Solid Edge part; units mm, degrees
sketch "Sketch1" plane through (0, 0, 0) normal (0, -1, 0) x (1, 0, 0)
  line L0 (-5.4714, -0.2002) -> (36.8286, -0.2002)
  line L1 (36.8286, -0.2002) -> (36.8286, 42.0998)
  line L2 (36.8286, 42.0998) -> (-5.4714, 42.0998)
  line L3 (-5.4714, 42.0998) -> (-5.4714, -0.2002)
extrude "Protrusion1" add sketch "Sketch1" against normal blind 10
sketch "Sketch2" plane through (15.6786, 0, 20.9498) normal (0, -1, 0) x (1, 0, 0)
  circle A0 centre (0, 0) radius 11
extrude "ProtrusiónExtruida_2" add sketch "Sketch2" along normal blind 2
chamfer "Chaflán_2" distance 5 angle 45 4 edges at (36.8286, 5, 42.0998) (36.8286, 5, -0.2002) (-5.4714, 5, -0.2002) (-5.4714, 5, 42.0998)
sketch "Sketch3" plane through (15.6786, -2, 20.9498) normal (0, -1, 0) x (1, 0, 0)
  circle A0 centre (0, 0) radius 4
  circle A1 centre (15.5, 15.5) radius 1.5
  circle A2 centre (-15.5, 15.5) radius 1.5
  circle A3 centre (-15.5, -15.5) radius 1.5
  circle A4 centre (15.5, -15.5) radius 1.5
extrude "VaciadoExtruido_2" cut sketch "Sketch3" against normal blind 7
sketch "Sketch4" plane through (15.6786, 5, 20.9498) normal (0, -1, 0) x (1, 0, 0)
  circle A0 centre (0, 0) radius 2.5
extrude "ProtrusiónExtruida_3" add sketch "Sketch4" along normal blind 29
sketch "Sketch5" plane through (15.6786, 10, 20.9498) normal (0, 1, 0) x (0, 0, -1)
  line L0 (-21, -21) -> (21, -21)
  line L1 (21, -21) -> (21, 21)
  line L2 (21, 21) -> (-21, 21)
  line L3 (-21, 21) -> (-21, -21)
extrude "ProtrusiónExtruida_4" add sketch "Sketch5" along normal blind 4
chamfer "Chaflán_9" distance 5 angle 45 4 edges at (-5.3214, 12, 41.9498) (36.6786, 12, 41.9498) (36.6786, 12, -0.0502) (-5.3214, 12, -0.0502)
sketch "Sketch6" plane through (15.6786, 14, 20.9498) normal (0, 1, 0) x (0, 0, -1)
  line L0 (21.15, -21.15) -> (-21.15, -21.15)
  line L1 (-21.15, -21.15) -> (-21.15, 21.15)
  line L2 (-21.15, 21.15) -> (21.15, 21.15)
  line L3 (21.15, 21.15) -> (21.15, -21.15)
extrude "ProtrusiónExtruida_5" add sketch "Sketch6" along normal blind 10
chamfer "Chaflán_10" distance 5 angle 45 4 edges at (36.8286, 19, 42.0998) (-5.4714, 19, 42.0998) (-5.4714, 19, -0.2002) (36.8286, 19, -0.2002)
sketch "Sketch7" plane through (15.6786, 24, 20.9498) normal (0, 1, 0) x (-1, 0, 0)
  circle A0 centre (0, 0) radius 4
  circle A1 centre (-15.5, 15.5) radius 2.25
  circle A2 centre (15.5, 15.5) radius 2.25
  circle A3 centre (15.5, -15.5) radius 2.25
  circle A4 centre (-15.5, -15.5) radius 2.25
extrude "VaciadoExtruido_3" cut sketch "Sketch7" against normal blind 5
Could you check a few things on this model? Use its own coordinates, in mm. A direction names the side the tool comes from. Round coordinates to 2 decimals unless told otherwise and drop trailing zeros. Write each loop counter-clockwise with the first axis right and the second up, starting at its lowest first coordinate (ties: lowest second). Pieces come first, ordered by that corner, then holes. Notation, with made-up numbers: M -12.75,30 L 0.25,30 A9 ccw 0.25,36 Z; hole C 25,-28 d7. An arc over 180 degrees is marked long. Write each question's results on one line, items separated by ' | '. Start each with the question number.
1. Imagine slicing it at B-B on x = 4. List the corners of the cut face in (y, z) for me.
2. I need wall thicknesses on L1, parallel to Y at x = 4, z = 23; L2, parallel to Y at x = 7.5, z = 14.5; L3, parallel to X at y = -1.5, z = 12.5. Which ranges of each line are inside material? Lowest first, please. Write a range as from..to.
3. Imagine slicing it at C-C on y = 2. List the corners of the cut face in (x, z) for me, and give its area (3 significant figures).
4. Imagine slicing it at D-D on z = 33. List the corners of the cut face in (x, y) for me.
5. On a 3-axis mill with a long thin cutter (end or side, diameter ignored), from which of +Z, -Z, +X, -X, +Y, -Y can I reach the whole of each face in a straight line? I mean faces 5 (the face through (-2.786, 11.972, 2.415)), 6 (the face through (18.63, 21.54, 23.65)), 7 (the face through (36.679, 12, 21)). Say none if no direction works.
6. Thinking about a two-plate mould opening in Z: for faces 1 (the face through (36.829, 19, 21)), 2 (the face through (34.36, 4.93, 2.33)), 3 (the face through (0, 5, 5)), 4 (the face through (16, 19, 21)), which applies, +Z half, -Z half, draft (parallel to the pull), parting line (faces both ways), or undercut?
7. I'm going to push flat-ended pins straight in: pin 1 Ø1.3 at (x, z) = (31, 35.5) entering from +Y; pin 2 Ø2.5 at (x, z) = (0.18, 5.45) entering from -Y; pin 3 Ø2.5 at (x, z) = (1, 36.5) entering from -Y. Where does each tip first touch, or does it pass through?
8. Imagine slicing it at A-A on y = 12.5. List the corners of the cut face in (x, z) for me, and give its area (3 significant figures).
Result sheet:
1) outline: M 0,-0.2 L 10,-0.2 L 10,-0.05 L 14,-0.05 L 14,-0.2 L 24,-0.2 L 24,42.1 L 14,42.1 L 14,41.95 L 10,41.95 L 10,42.1 L 0,42.1 Z
2) L1: y = 0..24 | L2: y = -2..24 | L3: x = 8.64..22.72
3) outline: M -5.47,4.8 L -0.47,-0.2 L 31.83,-0.2 L 36.83,4.8 L 36.83,37.1 L 31.83,42.1 L -0.47,42.1 L -5.47,37.1 Z; C 15.68,20.95 d5; hole C 0.18,5.45 d3; hole C 0.18,36.45 d3; hole C 15.68,20.95 d8; hole C 31.18,5.45 d3; hole C 31.18,36.45 d3 | area: 1,680 mm^2
4) outline: M -5.47,0 L 36.83,0 L 36.83,10 L 36.68,10 L 36.68,14 L 36.83,14 L 36.83,24 L -5.47,24 L -5.47,14 L -5.32,14 L -5.32,10 L -5.47,10 Z
5) face 5: -Z, -X | face 6: +Y | face 7: +Z, -Z, +X
6) face 1: draft | face 2: -Z half | face 3: undercut | face 4: undercut
7) pin 1: stops at y = 19 | pin 2: stops at y = 5 | pin 3: stops at y = 0
8) outline: M -5.32,4.95 L -0.32,-0.05 L 31.68,-0.05 L 36.68,4.95 L 36.68,36.95 L 31.68,41.95 L -0.32,41.95 L -5.32,36.95 Z | area: 1,710 mm^2
